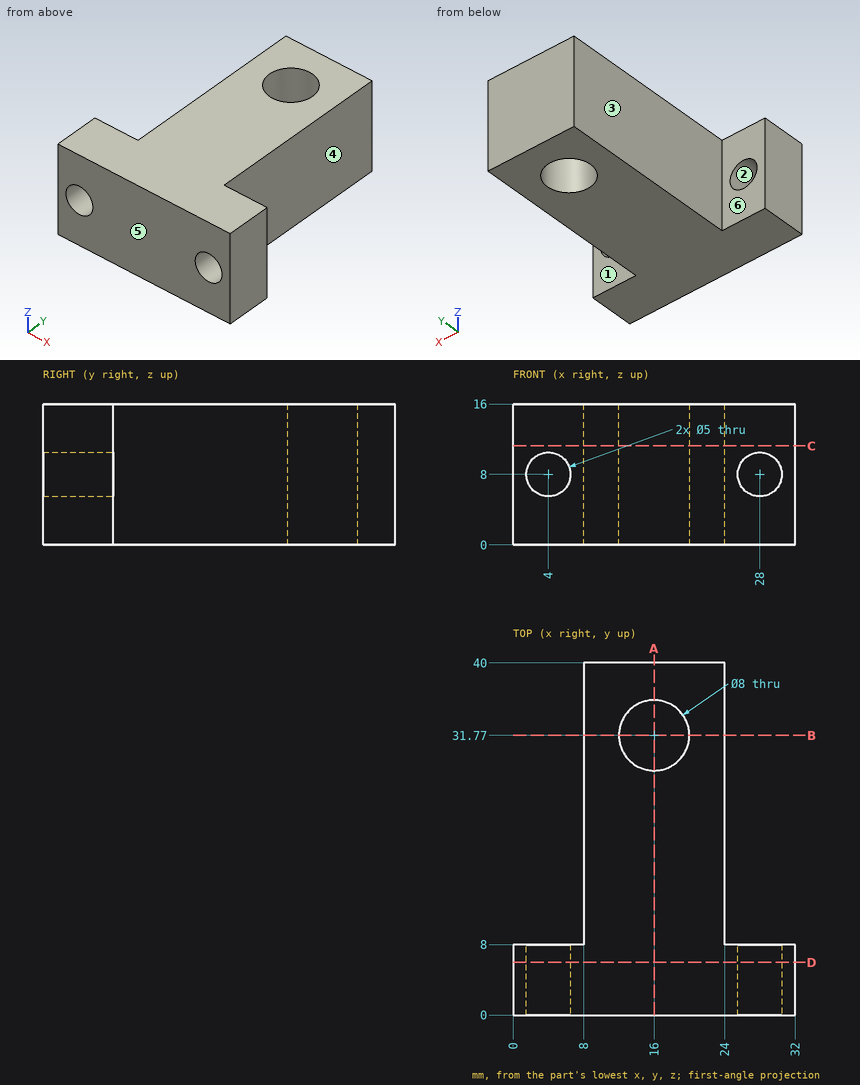
Geometry check sheet. Reference: drawing and pictorial views, mm from the part's lowest x, y, z. A direction names the side the tool comes from. Coordinates: 2 decimals unless noted, no trailing zeros. Order: outer loops, then holes, each group sorted by start corner. A loop starts at its lowest first (then second) coordinate and runs counter-clockwise, first axis right, second up.
Item 1: Tool access check on the marked faces 4, 5 and 6. Record the directions out of +Z, -Z, +X, -X, +Y, -Y that give a thin tool (end or side, any length) a straight path to the whole face; none if there is none.
Item 2: Section check D-D (y = 6). Enter the section's corners in (x, z).
Item 3: Depth check by flat-ended pin: pin 1 (5 mm diameter, centred on y = 21.5, z = 6.5, fed in from +X); pin 2 (4.5 mm diameter, centred on x = 4, z = 8, fed in from +Y); pin 3 (2.5 mm diameter, centred on x = 27, z = 10.5, fed in from +Y). Enter the tip coordinate at first touch or a pass-through.
Item 4: Mould release check, pull along X, two halves, no side actions. Record for the marked faces 1, 2 and 3: released by +X, released by -X, zero draft, split by the parting line, or undercut.
Item 5: Section check C-C (z = 11.25). Enter the section's corners in (x, y), plus the area to 3 significant figures.
Item 6: Section check A-A (x = 16). Enter the section's corners in (y, z), plus the area to 3 significant figures.
Item 7: Section check B-B (y = 31.77). Enter the section's corners in (x, z).
Item 8: Scan lines: line 1 along X through (y, z) = (3.5, 8); line 2 along Z through (x, y) = (28, 2.5); line 3 along X through (y, z) = (6.5, 9.75). Record each from-to range of solid material in increasing order.
Check sheet entries:
1. face 4: +Z, -Z, +X, +Y
1. face 5: +Z, -Z, +X, -X, -Y
1. face 6: +Z, -Z, -X, +Y
2. outline: (0, 0) - (32, 0) - (32, 16) - (0, 16) - close; hole circle Ø5 at (4, 8); hole circle Ø5 at (28, 8)
3. pin 1: stops at x = 24
3. pin 2: passes through
3. pin 3: stops at y = 8
4. face 1: zero draft
4. face 2: undercut
4. face 3: released by -X
5. outline: (0, 0) - (32, 0) - (32, 8) - (24, 8) - (24, 40) - (8, 40) - (8, 8) - (0, 8) - close; hole circle Ø8 at (16, 31.77)
5. area: 718 mm2
6. outline: (0, 0) - (27.77, 0) - (27.77, 16) - (0, 16) - close; (35.77, 0) - (40, 0) - (40, 16) - (35.77, 16) - close
6. area: 512 mm2
7. outline: (8, 0) - (12, 0) - (12, 16) - (8, 16) - close; (20, 0) - (24, 0) - (24, 16) - (20, 16) - close
8. line 1: x = 0 to 1.5, 6.5 to 25.5, 30.5 to 32
8. line 2: z = 0 to 5.5, 10.5 to 16
8. line 3: x = 0 to 2.21, 5.79 to 26.21, 29.79 to 32
